```python
from build123d import *

# Parameters (mm, degrees)
SKETCH1_W                                       = 25.4
SKETCH1_H                                       = 50.8
SKETCH1_W_2                                     = 19.05
SKETCH1_H_2                                     = 44.45
EXTRUDE_THIN1_DEPTH                             = 527.05
F_10_CLEARANCE_HOLE1_D                          = 5.1054
F_1_8_0_13_DIAMETER_HOLE1_D                     = 3.302
F_1_8_0_13_DIAMETER_HOLE1_DEPTH                 = 3.175
F_1_8_0_13_DIAMETER_HOLE2_D                     = 3.302
F_1_8_0_13_DIAMETER_HOLE2_DEPTH                 = 3.175
F_1_4_CLEARANCE_HOLE1_D                         = 6.7564
F_1_4_CLEARANCE_HOLE1_DEPTH                     = 10.7188
F_1_4_CLEARANCE_HOLE1_TIP                       = 2.029827343
CBORE_FOR_10_SOCKET_HEAD_CAP_SCREW1_D           = 5.1054
CBORE_FOR_10_SOCKET_HEAD_CAP_SCREW1_CBORE_D     = 9.525
CBORE_FOR_10_SOCKET_HEAD_CAP_SCREW1_CBORE_DEPTH = 8.001


with BuildPart() as part:
    # Sketch1 → Extrude-Thin1 (new body)
    with BuildSketch(Plane.XY):
        Rectangle(SKETCH1_W, SKETCH1_H)
        Rectangle(SKETCH1_W_2, SKETCH1_H_2, mode=Mode.SUBTRACT)
    extrude(amount=EXTRUDE_THIN1_DEPTH)

    # #10 Clearance Hole1 (through all)
    with Locations(Plane(origin=(0, 25.4, 0), x_dir=(1, 0, 0), z_dir=(0, 1, 0))):
        with Locations((0, -520.7), (0, -495.3), (0, -469.9), (0, -6.35), (0, -31.75), (0, -57.15)):
            Hole(F_10_CLEARANCE_HOLE1_D / 2)

    # 1/8 (0.13) Diameter Hole1
    with Locations(Plane(origin=(0, -25.4, 0), x_dir=(-1, 0, 0), z_dir=(0, -1, 0))):
        with Locations((3.175, -451.358), (-3.175, -425.958), (3.175, -400.558), (-3.175, -375.158), (3.175, -349.758), (3.175, -298.958), (3.175, -248.158), (-3.175, -222.758), (3.175, -197.358), (-3.175, -171.958), (3.175, -146.558), (-3.175, -121.158), (-3.175, -70.358), (-3.175, -324.358), (-3.175, -273.558), (3.175, -95.758)):
            Hole(F_1_8_0_13_DIAMETER_HOLE1_D / 2, depth=F_1_8_0_13_DIAMETER_HOLE1_DEPTH)

    # 1/8 (0.13) Diameter Hole2
    with Locations(Plane(origin=(0, 25.4, 0), x_dir=(1, 0, 0), z_dir=(0, 1, 0))):
        with Locations((4.92125, -313.055), (4.92125, -280.035), (4.92125, -247.015), (4.92125, -213.995)):
            Hole(F_1_8_0_13_DIAMETER_HOLE2_D / 2, depth=F_1_8_0_13_DIAMETER_HOLE2_DEPTH)

    # 1/4 Clearance Hole1
    with Locations(Plane(origin=(0, 25.4, 0), x_dir=(1, 0, 0), z_dir=(0, 1, 0))):
        with Locations((-3.175, -146.05), (-3.175, -381)):
            Hole(F_1_4_CLEARANCE_HOLE1_D / 2, depth=F_1_4_CLEARANCE_HOLE1_DEPTH)
            with Locations((0, 0, -(F_1_4_CLEARANCE_HOLE1_DEPTH + F_1_4_CLEARANCE_HOLE1_TIP / 2))):  # 118° drill point
                Cone(0, F_1_4_CLEARANCE_HOLE1_D / 2, F_1_4_CLEARANCE_HOLE1_TIP, mode=Mode.SUBTRACT)

    # CBORE for #10 Socket Head Cap Screw1 (through all)
    with Locations(Plane(origin=(12.7, 0, 0), x_dir=(0, 0, -1), z_dir=(1, 0, 0))):
        with Locations((-111.125, -12.7), (-123.825, -12.7), (-136.525, -12.7), (-390.525, -12.7), (-415.925, -12.7), (-403.225, -12.7)):
            CounterBoreHole(CBORE_FOR_10_SOCKET_HEAD_CAP_SCREW1_D / 2, CBORE_FOR_10_SOCKET_HEAD_CAP_SCREW1_CBORE_D / 2, CBORE_FOR_10_SOCKET_HEAD_CAP_SCREW1_CBORE_DEPTH)


solid = part.part
```
CAD build for the part. Positions are in the model's coordinates, mm. A direction names the side the tool comes from. Round coordinates to 2 decimals unless told otherwise and drop trailing zeros. Order: outer loops, then holes, each group sorted by start corner. A loop starts at its lowest first (then second) coordinate and runs counter-clockwise, first axis right, second up. Notation, with made-up numbers: (0, 8.25) - (38, 8.25) arc R23 cw to (38, 27.25) - close; hole circle Ø8 at (53, 51). An arc over 180 degrees is marked (long way). Answer as CSV lines item,"result". Start each with the question number.
1. Saw through at A-A, the plane y = 3. Write the cut outline in (x, z) (3 decimals), and give its area (3 significant figures).
2. Drill centre lines: L1, parallel to X at y = 24, z = 57.15; L2, parallel to X at y = -1, z = 196 (3 decimals); L3, parallel to Y at x = 8.5, z = 152.5 (3 decimals). Where is each one in solid material? Low to high. Write a range as [from, to].
3. Saw through at B-B, the plane z = 187. Write the cut outline in (x, y) (3 decimals).
4. Pull direction X, two halves, no side cores. Call faces 1 (the face through (-12.7, 0, 260)), 2 (the face through (11.135, -11.269, 398.682)), 3 (the face through (0, 22.225, 260)): +X half, -X half, draft (parallel to the pull), parting line (faces both ways), or undercut.
5. Tool access for faces 4 (the face through (-10, -2, 527.05)), 5 (the face through (0, -22.225, 260)), 6 (the face through (11.135, -12.491, 141.283)): list every direction of +Z, -Z, +X, -X, +Y, -Y with a clear straight run to the whole face (end or side of a thin tool).
Model answer:
1,outline,"(-12.7, 0) - (-9.525, 0) - (-9.525, 527.05) - (-12.7, 527.05) - close; (9.525, 0) - (12.7, 0) - (12.7, 527.05) - (9.525, 527.05) - close"
1,area,"3,350 mm²"
2,L1,"x = [-12.7, -2.55], [2.55, 12.7]"
2,L2,"x = [-12.7, -9.525], [9.525, 12.7]"
2,L3,"y = [-25.4, -22.225], [22.225, 25.4]"
3,outline,"(-12.7, -25.4) - (12.7, -25.4) - (12.7, 25.4) - (-12.7, 25.4) - close; hole (-9.525, -22.225) - (9.525, -22.225) - (9.525, 22.225) - (-9.525, 22.225) - close"
4,face 1,"-X half"
4,face 2,"draft"
4,face 3,"undercut"
5,face 4,"+Z, +X, -X, +Y, -Y"
5,face 5,"+Z, -Z"
5,face 6,"+X"
